Here's how the part is built. I have some questions about the finished solid (model axes, mm). Face numbers are marked on the shaded views. A direction names the side the tool comes from. Coordinates: 2 decimals unless noted, no trailing zeros. Write each loop counter-clockwise with the first axis right and the second up, starting at its lowest first coordinate (ties: lowest second). Pieces come first, ordered by that corner, then holes. Notation, with made-up numbers: M 36,-33 L 74,-33 A26 ccw 74,2 Z; hole C 59,-39 d8. An arc over 180 degrees is marked long. Use a Markdown table: item, result.
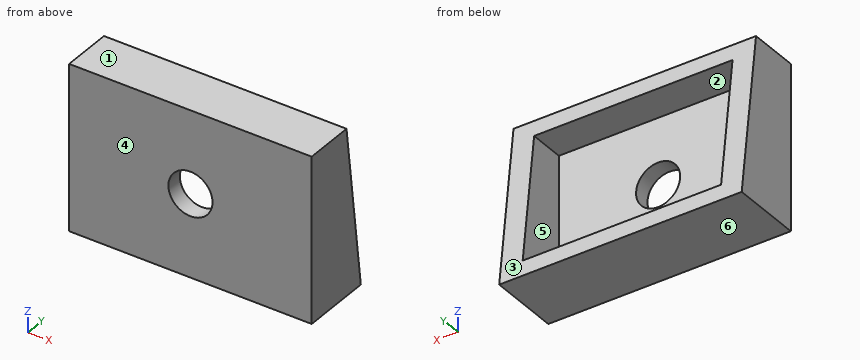
```python
from build123d import *

# Parameters (mm, degrees)
SKETCH2_W               = 22
SKETCH2_H               = 15
BOSS_EXTRUDE1_DEPTH     = 8
CUT_EXTRUDE2_DEPTH      = 27.248809497
CUT_EXTRUDE2_DEPTH_BACK = 27.248809497
SKETCH7_W               = 12
SKETCH7_H               = 5.260019913
CUT_EXTRUDE3_DEPTH      = 18
CUT_EXTRUDE4_DEPTH      = 28.082872227
CUT_EXTRUDE4_DEPTH_BACK = 28.082872227
SKETCH9_R               = 2


with BuildPart() as part:
    # Sketch2 → Boss-Extrude1 (new body)
    with BuildSketch(Plane(origin=(0, 0, 0), x_dir=(1, 0, 0), z_dir=(0, 1, 0))):
        with Locations((11, 7.5)):
            Rectangle(SKETCH2_W, SKETCH2_H)
    extrude(amount=BOSS_EXTRUDE1_DEPTH)

    # Sketch6 → Cut-Extrude2 (cut, two sides: drawn at the far end of the back side and taken through both)
    with BuildSketch(Plane(origin=(2, 0, 0), x_dir=(0, 0, -1), z_dir=(1, 0, 0)).offset(-CUT_EXTRUDE2_DEPTH_BACK)):
        Polygon((-0.545340916, 4.5), (15.415577352, 6.5), (15.415577352, 8.571331794), (-0.545340916, 8.571331794), align=None)
    extrude(amount=CUT_EXTRUDE2_DEPTH + CUT_EXTRUDE2_DEPTH_BACK, mode=Mode.SUBTRACT)

    # Sketch7 → Cut-Extrude3 (cut)
    with BuildSketch(Plane(origin=(2, 0, 0), x_dir=(0, 0, -1), z_dir=(1, 0, 0))):
        with Locations((7.5, 4.130009957)):
            Rectangle(SKETCH7_W, SKETCH7_H)
    extrude(amount=CUT_EXTRUDE3_DEPTH, mode=Mode.SUBTRACT)

    # Sketch9 → Cut-Extrude4 (cut, two sides: drawn at the far end of the back side and taken through both)
    with BuildSketch(Plane(origin=(0, 1.5, 0), x_dir=(1, 0, 0), z_dir=(0, 1, 0)).offset(-CUT_EXTRUDE4_DEPTH_BACK)):
        with Locations(Location((11, 7.5, 0), (0, 0, 270))):
            Circle(SKETCH9_R)
    extrude(amount=CUT_EXTRUDE4_DEPTH + CUT_EXTRUDE4_DEPTH_BACK, mode=Mode.SUBTRACT)


solid = part.part
```
1. Suppose I cut it at C-C on y = 3.25. Write out the boundary of the cut face in (x, z), and give its area (3 significant figures).
Answers follow:
| item | result |
|---|---|
| outline | M 0,-15 L 22,-15 L 22,0 L 0,0 Z; hole M 2,-13.5 L 20,-13.5 L 20,-1.5 L 2,-1.5 Z |
| area | 114 mm2 |
2. Which directions (+Z, -Z, +X, -X, +Y, -Y) give clear straight access to the entire face, cutting with the end or side of a thin tool? Please do the marked faces 1 and 2.
Answers follow:
| item | result |
|---|---|
| face 1 | +Z, +X, -X, +Y, -Y |
| face 2 | +Y |
3. Suppose I cut it at B-B on z = -6.25. Write out the boundary of the cut face in (x, y), and give its area (3 significant figures).
Answers follow:
| item | result |
|---|---|
| outline | M 0,0 L 9.44,0 L 9.44,1.5 L 2,1.5 L 2,5.35 L 0,5.35 Z; M 12.56,0 L 22,0 L 22,5.35 L 20,5.35 L 20,1.5 L 12.56,1.5 Z |
| area | 43.7 mm2 |
4. I need wall thicknesses on probe 1 along Z at (x, y) = (11, 0.4); probe 2 along X at (y, z) = (3, -8.5); probe 3 along Z at (x, y) = (10.25, 4). Which ranges of each line are inside material? Lowest first, please.
Answers follow:
| item | result |
|---|---|
| probe 1 | z = -15 to -9.5, -5.5 to 0 |
| probe 2 | x = 0 to 2, 20 to 22 |
| probe 3 | z = -15 to -13.5, -1.5 to 0 |
5. Suppose I cut it at D-D on x = 7.75. Write out the boundary of the cut face in (y, z).
Answers follow:
| item | result |
|---|---|
| outline | M 0,-15 L 6.45,-15 L 6.26,-13.5 L 1.5,-13.5 L 1.5,-1.5 L 4.76,-1.5 L 4.57,0 L 0,0 Z |
6. We'd pull the mould along Z, two halves only. Please class the marked faces 3, 4, 5 and 6: +Z half, -Z half, draft (parallel to the pull), parting line (faces both ways), or undercut.
Answers follow:
| item | result |
|---|---|
| face 3 | +Z half |
| face 4 | draft |
| face 5 | undercut |
| face 6 | -Z half |
7. Will this pin go through, and if not, where does the flat tip stop? pin 1 Ø5 at (x, z) = (11, -7.5) entering from +Y.
Answers follow:
| item | result |
|---|---|
| pin 1 | stops at y = 1.5 |
8. Suppose I cut it at A-A on x = 11. Write out the boundary of the cut face in (y, z).
Answers follow:
| item | result |
|---|---|
| outline | M 0,-15 L 6.45,-15 L 6.26,-13.5 L 1.5,-13.5 L 1.5,-9.5 L 0,-9.5 Z; M 0,-5.5 L 1.5,-5.5 L 1.5,-1.5 L 4.76,-1.5 L 4.57,0 L 0,0 Z |
